Print and shaded views of the part. All mm, measured from the part's lowest x, y and z. A direction names the side the tool comes from. Coordinates: 2 decimals unless noted, no trailing zeros. Loops run counter-clockwise (first coordinate to the right, second up) from the corner with the lowest first, then second, coordinate; pieces in that order, holes last. Notation, with made-up numbers: M 31.5,-3 L 59.5,-3 A18 ccw 59.5,2 Z; hole C 42,11.25 d4. An arc over 180 degrees is marked long. Answer as CSV lines item,"result". Start each with the question number.
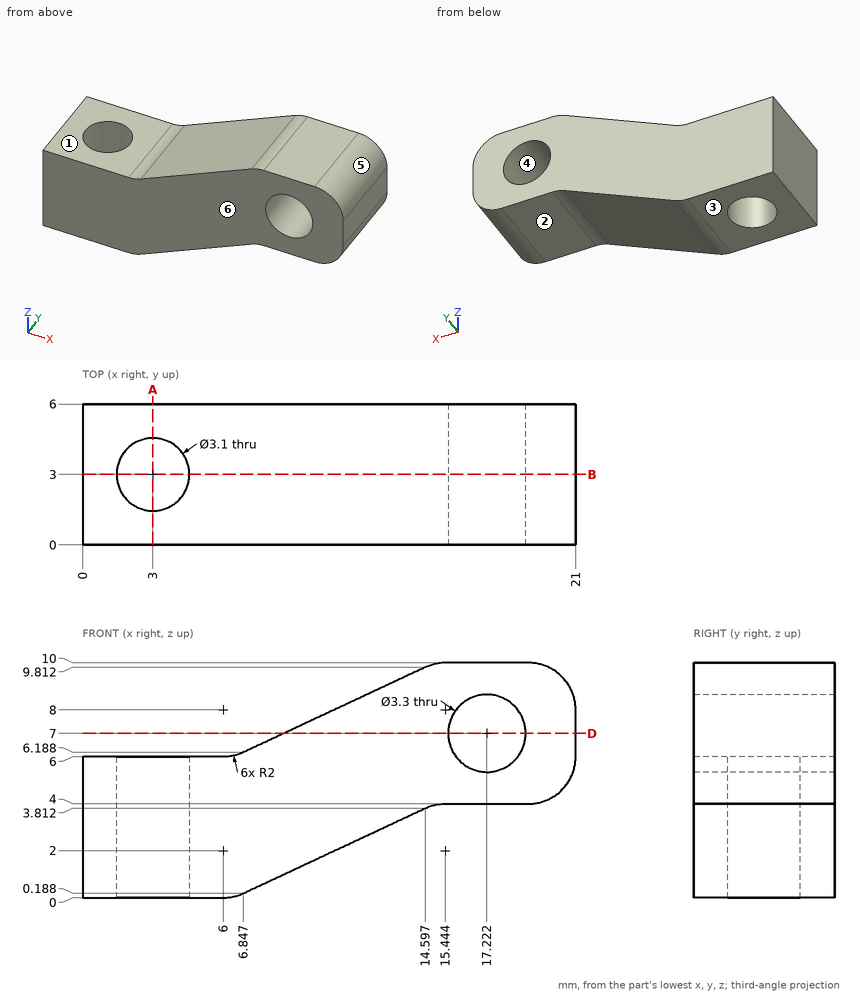
Q1. Flat gauge pins, fed straight in: P1, Ø3, axis at x = 17.22, z = 7, coming from the -Y side; P2, Ø2, axis at x = 2, y = 4, coming from the +Z side. Where does each tip first touch, or does it go through?
Q2. Wall check: L1, parallel to Y at x = 3, z = 4.35; L2, parallel to Z at x = 4.75, y = 4.25; L3, parallel to Z at x = 17.5, y = 3.6. Give the ranges that are in metal, low to high.
Q3. Slice it at D-D, the plane z = 7. Write the cut outline in (x, y).
Q4. Slice it at B-B, the plane y = 3. State how many separate pieces and enclosed holes the cut face has.
Q5. Tool access for the marked faces 1, 2 and 3: list every direction of +Z, -Z, +X, -X, +Y, -Y with a clear straight run to the whole face (end or side of a thin tool).
Q6. Slice it at A-A, the plane x = 3. Write the cut outline in (y, z).
Q7. Two-plate mould, pull along X, no slides. Class the marked faces 4, 5 and 6: +X half, -X half, draft (parallel to the pull), parting line (faces both ways), or undercut.
Solved:
1,P1,"passes through"
1,P2,"stops at z = 6"
2,L1,"y = 0 to 1.45, 4.55 to 6"
2,L2,"z = 0 to 6"
2,L3,"z = 4 to 5.37, 8.63 to 10"
3,outline,"M 8.58,0 L 15.57,0 L 15.57,6 L 8.58,6 Z; M 18.87,0 L 21,0 L 21,6 L 18.87,6 Z"
4,separate pieces,"2"
4,enclosed holes,"1"
5,face 1,"+Z, -X, +Y, -Y"
5,face 2,"-Z, +X, +Y, -Y"
5,face 3,"-Z, +X, -X, +Y, -Y"
6,outline,"M 0,0 L 1.45,0 L 1.45,6 L 0,6 Z; M 4.55,0 L 6,0 L 6,6 L 4.55,6 Z"
7,face 4,"undercut"
7,face 5,"+X half"
7,face 6,"draft"
